The model under review builds one solid part; all positions refer to its coordinate system, in mm. A direction names the side the tool comes from. Round coordinates to 2 decimals unless told otherwise and drop trailing zeros. Write each loop counter-clockwise with the first axis right and the second up, starting at its lowest first coordinate (ties: lowest second). Pieces come first, ordered by that corner, then holes. Notation, with made-up numbers: (83.5, -17) -> (106.5, -17) arc R24 cw to (106.5, -1) -> close; hole circle Ø3 at (23, 3). An arc over 180 degrees is marked (long way). Return JSON: item names as keys, results as strings. Group by question number.
1. Take a section at B-B, the plane z = -35. Write out the cut boundary in (x, y), then the cut area to 3 significant figures.
2. For line 1 along Y through (x, z) = (15.75, -29); line 2 along Y through (x, z) = (1.75, -21); line 3 along Z through (x, y) = (5, 23.5), list the stretches that pass through material, from the lowest coordinate up. Write a range as from..to.
3. Take a section at A-A, the plane x = 6. Write out the cut boundary in (y, z).
4. Tool access review of faces 1 (the flat face through (10, 30.48, -44)), 2 (the flat face through (10, 36, 0)), 3 (the cylindrical face through (9.68, 40.7, -23.73)), 4 (the flat face through (10, 27.178, -44)): name each direction out of +Z, -Z, +X, -X, +Y, -Y from which nothing blocks a thin tool from reaching the whole face with its end or side.
5. Take a section at D-D, the plane y = 33. Write out the cut boundary in (x, z), then the cut area to 3 significant figures.
6. Take a section at C-C, the plane x = 11. Write out the cut boundary in (y, z).
7. Clearance check with flat-ended pins moving along their axes: P1, Ø8, axis at x = 9, z = 5, coming from the +Y side; P2, Ø10, axis at x = 6, y = 36.5, coming from the -Z side; P3, Ø10, axis at x = 16.5, y = 16, coming from the +Z side. State where each tip first meets the part, or that it passes through.
from build123d import *

# Parameters (mm, degrees)
BOSS_EXTRUDE1_DEPTH = 19.939
SKETCH2_R           = 2.97815
BOSS_EXTRUDE2_DEPTH = 5.08
SKETCH3_R           = 6.477
BOSS_EXTRUDE3_DEPTH = 0.635
SKETCH4_R           = 2.2606
CUT_EXTRUDE1_DEPTH  = 60.674033694


with BuildPart() as part:
    # Sketch1 → Boss-Extrude1 (new body)
    with BuildSketch(Plane(origin=(0, 0, 0), x_dir=(0, 0, -1), z_dir=(1, 0, 0))):
        Polygon((0, 0), (40.1066, 0), (40.1066, 27.178), (47.2694, 27.178), (47.2694, 30.48), (40.1066, 30.48), (40.1066, 40.386), (0, 40.386), (0, 30.48), (-7.1628, 30.48), (-7.1628, 27.178), (0, 27.178), align=None)
    extrude(amount=BOSS_EXTRUDE1_DEPTH)

    # Sketch2 → Boss-Extrude2 (add)
    with BuildSketch(Plane(origin=(0, 40.386, 0), x_dir=(1, 0, 0), z_dir=(0, 1, 0))):
        with Locations(Location((9.9695, 30.2006, 0), (0, 0, 90))):
            Circle(SKETCH2_R)
    extrude(amount=BOSS_EXTRUDE2_DEPTH)

    # Sketch3 → Boss-Extrude3 (add)
    with BuildSketch(Plane(origin=(0, 40.386, 0), x_dir=(1, 0, 0), z_dir=(0, 1, 0))):
        with Locations(Location((9.9695, 30.2006, 0), (0, 0, 90))):
            Circle(SKETCH3_R)
    extrude(amount=BOSS_EXTRUDE3_DEPTH)

    # Sketch4 → Cut-Extrude1 (cut, through all)
    with BuildSketch(Plane(origin=(0, 30.48, 0), x_dir=(1, 0, 0), z_dir=(0, 1, 0))):
        with Locations(Location((5.0419, 44.1833, 0), (0, 0, 270))):
            Circle(SKETCH4_R)
        with Locations(Location((14.8971, 44.1833, 0), (0, 0, 270))):
            Circle(SKETCH4_R)
        with Locations(Location((14.8971, -4.0767, 0), (0, 0, 270))):
            Circle(SKETCH4_R)
        with Locations(Location((5.0419, -4.0767, 0), (0, 0, 270))):
            Circle(SKETCH4_R)
    extrude(amount=-CUT_EXTRUDE1_DEPTH, mode=Mode.SUBTRACT)


solid = part.part
Output:
{
 "1": {"outline": "(0, 0) -> (19.94, 0) -> (19.94, 40.39) -> (14.32, 40.39) -> (14.32, 41.02) -> (5.62, 41.02) -> (5.62, 40.39) -> (0, 40.39) -> close", "area": "811 mm^2"},
 "2": {"line 1": "y = 0..41.02", "line 2": "y = 0..40.39", "line 3": "z = -40.11..0"},
 "3": {"outline": "(0, -40.11) -> (27.18, -40.11) -> (27.18, -42.14) -> (30.48, -42.14) -> (30.48, -40.11) -> (40.39, -40.11) -> (40.39, -35.32) -> (41.02, -35.32) -> (41.02, -25.08) -> (40.39, -25.08) -> (40.39, 0) -> (30.48, 0) -> (30.48, 2.03) -> (27.18, 2.03) -> (27.18, 0) -> (0, 0) -> close; (27.18, -47.27) -> (30.48, -47.27) -> (30.48, -46.23) -> (27.18, -46.23) -> close; (27.18, 6.12) -> (30.48, 6.12) -> (30.48, 7.16) -> (27.18, 7.16) -> close"},
 "4": {"face 1": "-Z, +X, -X, +Y", "face 2": "+Z, +X, -X, +Y", "face 3": "+Y", "face 4": "-Z, +X, -X, -Y"},
 "5": {"outline": "(0, -40.11) -> (19.94, -40.11) -> (19.94, 0) -> (0, 0) -> close", "area": "800 mm^2"},
 "6": {"outline": "(0, -40.11) -> (27.18, -40.11) -> (27.18, -47.27) -> (30.48, -47.27) -> (30.48, -40.11) -> (40.39, -40.11) -> (40.39, -36.6) -> (41.02, -36.6) -> (41.02, -32.99) -> (45.47, -32.99) -> (45.47, -27.41) -> (41.02, -27.41) -> (41.02, -23.81) -> (40.39, -23.81) -> (40.39, 0) -> (30.48, 0) -> (30.48, 7.16) -> (27.18, 7.16) -> (27.18, 0) -> (0, 0) -> close"},
 "7": {"P1": "stops at y = 30.48", "P2": "stops at z = -40.11", "P3": "stops at z = 0"}
}
